```python
from build123d import *

# Parameters (mm, degrees)
BOSS_EXTRUDE1_DEPTH = 2.5
SHELL1_START        = -1.5
SHELL1_DEPTH        = 3
BOSS_EXTRUDE2_START = 2
BOSS_EXTRUDE2_DEPTH = 2
SKETCH4_W           = 30
SKETCH4_H           = 3
CUT_EXTRUDE1_DEPTH  = 100


# Read off the part's stored shape, not the designer's step: Shell1
with BuildPart() as part:
    # Sketch1 → Boss-Extrude1 (new, symmetric)
    with BuildSketch(Plane.XY):
        with BuildLine():
            ThreePointArc((-50.662558564, 50), (-52.076772126, 50.585786438), (-52.662558564, 52))
            Line((-52.662558564, 52), (-52.662558564, 53.937975118))
            ThreePointArc((-52.662558564, 53.937975118), (-52.498112524, 54.732167576), (-52.031816903, 55.395758229))
            ThreePointArc((-52.031816903, 55.395758229), (0, 76), (52.031816903, 55.395758229))
            ThreePointArc((52.031816903, 55.395758229), (52.498112524, 54.732167576), (52.662558564, 53.937975118))
            Line((52.662558564, 53.937975118), (52.662558564, 52))
            ThreePointArc((52.662558564, 52), (52.076772126, 50.585786438), (50.662558564, 50))
            Line((50.662558564, 50), (48.989794856, 50))
            ThreePointArc((48.989794856, 50), (0, 70), (-48.989794856, 50))
            Line((-48.989794856, 50), (-50.662558564, 50))
        make_face()
        with BuildLine():
            ThreePointArc((4.302180061, 56), (5.456880599, 55.632993162), (6.187798144, 54.666666667))
            ThreePointArc((6.187798144, 54.666666667), (8.029260752, 52.496291392), (10.847853752, 52.1))
            ThreePointArc((10.847853752, 52.1), (15.425940788, 52.068491802), (19.510205144, 50))
            Line((19.510205144, 50), (24.864501465, 50))
            ThreePointArc((24.864501465, 50), (25.78632175, 50.22510638), (26.500634408, 50.849752638))
            ThreePointArc((26.500634408, 50.849752638), (31, 53.186572392), (35.499365592, 50.849752638))
            ThreePointArc((35.499365592, 50.849752638), (36.21367825, 50.22510638), (37.135498535, 50))
            Line((37.135498535, 50), (48.989794856, 50))
            ThreePointArc((48.989794856, 50), (0, 70), (-48.989794856, 50))
            Line((-48.989794856, 50), (-37.135498535, 50))
            ThreePointArc((-37.135498535, 50), (-36.21367825, 50.22510638), (-35.499365592, 50.849752638))
            ThreePointArc((-35.499365592, 50.849752638), (-31, 53.186572392), (-26.500634408, 50.849752638))
            ThreePointArc((-26.500634408, 50.849752638), (-25.78632175, 50.22510638), (-24.864501465, 50))
            Line((-24.864501465, 50), (-19.510205144, 50))
            ThreePointArc((-19.510205144, 50), (-15.425940788, 52.068491802), (-10.847853752, 52.1))
            ThreePointArc((-10.847853752, 52.1), (-8.029260752, 52.496291392), (-6.187798144, 54.666666667))
            ThreePointArc((-6.187798144, 54.666666667), (-5.456880599, 55.632993162), (-4.302180061, 56))
            Line((-4.302180061, 56), (4.302180061, 56))
        make_face()
    extrude(amount=BOSS_EXTRUDE1_DEPTH, both=True)

    # Shell1 outline → Shell1 (cut)
    with BuildSketch(Plane.XY.offset(SHELL1_START)):
        with BuildLine():
            Line((37.135498535, 50), (50.662558564, 50))
            Line((50.662558564, 50), (50.662558564, 51))
            ThreePointArc((50.662558564, 51), (51.369665345, 51.292893219), (51.662558564, 52))
            Line((51.662558564, 52), (51.662558564, 53.937975118))
            ThreePointArc((51.662558564, 53.937975118), (51.580335544, 54.335071347), (51.347187733, 54.666866673))
            ThreePointArc((51.347187733, 54.666866673), (0, 75), (-51.347187733, 54.666866673))
            ThreePointArc((-51.347187733, 54.666866673), (-51.580335544, 54.335071347), (-51.662558564, 53.937975118))
            Line((-51.662558564, 53.937975118), (-51.662558564, 52))
            ThreePointArc((-51.662558564, 52), (-51.369665345, 51.292893219), (-50.662558564, 51))
            Line((-50.662558564, 51), (-50.662558564, 50))
            Line((-50.662558564, 50), (-37.135498535, 50))
            ThreePointArc((-37.135498535, 50), (-36.21367825, 50.22510638), (-35.499365592, 50.849752638))
            ThreePointArc((-35.499365592, 50.849752638), (-31, 53.186572392), (-26.500634408, 50.849752638))
            ThreePointArc((-26.500634408, 50.849752638), (-25.78632175, 50.22510638), (-24.864501465, 50))
            Line((-24.864501465, 50), (-19.510205144, 50))
            ThreePointArc((-19.510205144, 50), (-15.425940787, 52.068491802), (-10.847853752, 52.1))
            ThreePointArc((-10.847853752, 52.1), (-8.029260752, 52.496291392), (-6.187798144, 54.666666667))
            ThreePointArc((-6.187798144, 54.666666667), (-5.456880599, 55.632993162), (-4.302180061, 56))
            Line((-4.302180061, 56), (4.302180061, 56))
            ThreePointArc((4.302180061, 56), (5.456880599, 55.632993162), (6.187798144, 54.666666667))
            ThreePointArc((6.187798144, 54.666666667), (8.029260752, 52.496291392), (10.847853752, 52.1))
            ThreePointArc((10.847853752, 52.1), (15.425940787, 52.068491802), (19.510205144, 50))
            Line((19.510205144, 50), (24.864501465, 50))
            ThreePointArc((24.864501465, 50), (25.78632175, 50.22510638), (26.500634408, 50.849752638))
            ThreePointArc((26.500634408, 50.849752638), (31, 53.186572392), (35.499365592, 50.849752638))
            ThreePointArc((35.499365592, 50.849752638), (36.21367825, 50.22510638), (37.135498535, 50))
        make_face()
    extrude(amount=SHELL1_DEPTH, mode=Mode.SUBTRACT)

    # Sketch3 → Boss-Extrude2 (add)
    with BuildSketch(Plane.XY.offset(2.5).offset(BOSS_EXTRUDE2_START)):
        with BuildLine():
            ThreePointArc((48.989794856, 50), (0, 70), (-48.989794856, 50))
            Line((-48.989794856, 50), (-37.135498535, 50))
            ThreePointArc((-37.135498535, 50), (-36.21367825, 50.22510638), (-35.499365592, 50.849752638))
            ThreePointArc((-35.499365592, 50.849752638), (-31, 53.186572392), (-26.500634408, 50.849752638))
            ThreePointArc((-26.500634408, 50.849752638), (-25.78632175, 50.22510638), (-24.864501465, 50))
            Line((-24.864501465, 50), (-19.510205144, 50))
            ThreePointArc((-19.510205144, 50), (-15.425940788, 52.068491802), (-10.847853752, 52.1))
            ThreePointArc((-10.847853752, 52.1), (-8.029260752, 52.496291392), (-6.187798144, 54.666666667))
            ThreePointArc((-6.187798144, 54.666666667), (-5.456880599, 55.632993162), (-4.302180061, 56))
            Line((-4.302180061, 56), (4.302180061, 56))
            ThreePointArc((4.302180061, 56), (5.456880599, 55.632993162), (6.187798144, 54.666666667))
            ThreePointArc((6.187798144, 54.666666667), (8.029260752, 52.496291392), (10.847853752, 52.1))
            ThreePointArc((10.847853752, 52.1), (15.425940788, 52.068491802), (19.510205144, 50))
            Line((19.510205144, 50), (24.864501465, 50))
            ThreePointArc((24.864501465, 50), (25.78632175, 50.22510638), (26.500634408, 50.849752638))
            ThreePointArc((26.500634408, 50.849752638), (31, 53.186572392), (35.499365592, 50.849752638))
            ThreePointArc((35.499365592, 50.849752638), (36.21367825, 50.22510638), (37.135498535, 50))
            Line((37.135498535, 50), (48.989794856, 50))
        make_face()
    extrude(amount=-BOSS_EXTRUDE2_DEPTH)

    # Sketch4 → Cut-Extrude1 (cut, symmetric)
    with BuildSketch(Plane(origin=(0, 0, 0), x_dir=(1, 0, 0), z_dir=(0, 1, 0))):
        with Locations((-20, 0)):
            Rectangle(SKETCH4_W, SKETCH4_H)
        with Locations((20, 0)):
            Rectangle(SKETCH4_W, SKETCH4_H)
    extrude(amount=CUT_EXTRUDE1_DEPTH, both=True, mode=Mode.SUBTRACT)


solid = part.part
```
The model under review builds one solid part; all positions refer to its coordinate system, in mm. A direction names the side the tool comes from. Coordinates: 2 decimals unless noted, no trailing zeros. Write each loop counter-clockwise with the first axis right and the second up, starting at its lowest first coordinate (ties: lowest second). Pieces come first, ordered by that corner, then holes. Notation, with made-up numbers: (16.25, 54) -> (55.25, 54) arc R15 ccw to (55.25, 58) -> close; hole circle Ø3 at (-32.75, -17). An arc over 180 degrees is marked (long way). One line per item, written item: value. Start each with the question number.
Q1. For faces 4 (the face through (0.76, 69.996, 3.514)), 5 (the face through (-44, 50, 3)), 6 (the face through (0, 56, 3)), 7 (the face through (-51.663, 53, 0)), 8 (the face through (-52.663, 53, 0)), list the 3-axis set-ups (+Z, -Z, +X, -X, +Y, -Y) from which the entire face can be reached by the end or side of a thin tool; tool diameter is ignored.
Q2. Add section B-B, the plane y = 68.75. Give the boundary of the cut face in (x, z).
Q3. The part is to be moulded in two halves that separate along Z. For faces 1 (the face through (52.09, 50.6, 0.04)), 2 (the face through (51.663, 53, 0)), 3 (the face through (-1, 60, 4.5)), say which applies: +Z half, -Z half, draft (parallel to the pull), parting line (faces both ways), or undercut.
Q4. Add section A-A, the plane z = -0.5. Give the boundary of the cut face in (x, y), then the cut area to 3 significant figures.
Q5. Add section D-D, the plane z = 3.5. Give the boundary of the cut face in (x, y), then the cut area to 3 significant figures.
Q6. Add section C-C, the plane x = 31. Give the boundary of the cut face in (y, z).
Q7. To check wall thickness, follow probe 1 along Z at (x, y) = (-27.5, 68); probe 2 along Z at (x, y) = (-16, 58.25); probe 3 along X at (y, z) = (61.75, -0.5). State the ranges of each line that lie inside material, in increasing order.
Q8. Clearance check with flat-ended pins moving along their axes: P1, Ø3, axis at x = 37, y = 70, coming from the -Z side; P2, Ø0.8, axis at y = 50.5, z = 0.5, coming from the -X side; P3, Ø0.8, axis at y = 75.5, z = 0, coming from the -X side; P4, Ø0.6, axis at y = 66.5, z = 0.5, coming from the +X side. State where each tip first meets the part, or that it passes through.
Response:
1. face 4: +Z, +Y
1. face 5: +Z, -Z, +X, -X, -Y
1. face 6: +Z, -Z, -Y
1. face 7: none
1. face 8: +Z, -Z, -X, +Y, -Y
2. outline: (-32.4, -2.5) -> (32.4, -2.5) -> (32.4, -1.5) -> (-32.4, -1.5) -> close; (-32.4, 1.5) -> (32.4, 1.5) -> (32.4, 2.5) -> (13.17, 2.5) -> (13.17, 4.5) -> (-13.17, 4.5) -> (-13.17, 2.5) -> (-32.4, 2.5) -> close
3. face 1: draft
3. face 2: undercut
3. face 3: +Z half
4. outline: (-52.66, 52) arc R2 ccw to (-50.66, 50) -> (-50.66, 51) arc R1 cw to (-51.66, 52) -> (-51.66, 53.94) arc R1 cw to (-51.35, 54.67) arc R75 cw to (-35, 66.33) -> (-35, 67.46) arc R76 ccw to (-52.03, 55.4) arc R2 ccw to (-52.66, 53.94) -> close; (-5, 74.83) arc R75 cw to (5, 74.83) -> (5, 75.84) arc R76 ccw to (-5, 75.84) -> close; (35, 66.33) arc R75 cw to (51.35, 54.67) arc R1 cw to (51.66, 53.94) -> (51.66, 52) arc R1 cw to (50.66, 51) -> (50.66, 50) arc R2 ccw to (52.66, 52) -> (52.66, 53.94) arc R2 ccw to (52.03, 55.4) arc R76 ccw to (35, 67.46) -> close
4. area: 62.1 mm²
5. outline: (-48.99, 50) -> (-37.14, 50) arc R2 ccw to (-35.5, 50.85) arc R5.5 cw to (-26.5, 50.85) arc R2 ccw to (-24.86, 50) -> (-19.51, 50) arc R10 cw to (-10.85, 52.1) arc R4 ccw to (-6.19, 54.67) arc R2 cw to (-4.3, 56) -> (4.3, 56) arc R2 cw to (6.19, 54.67) arc R4 ccw to (10.85, 52.1) arc R10 cw to (19.51, 50) -> (24.86, 50) arc R2 ccw to (26.5, 50.85) arc R5.5 cw to (35.5, 50.85) arc R2 ccw to (37.14, 50) -> (48.99, 50) arc R70 ccw to start
5. area: 1,170 mm²
6. outline: (53.19, -2.5) -> (69.39, -2.5) -> (69.39, -1.5) -> (53.19, -1.5) -> close; (53.19, 1.5) -> (69.39, 1.5) -> (69.39, 2.5) -> (62.76, 2.5) -> (62.76, 4.5) -> (53.19, 4.5) -> close
7. probe 1: -2.5 to -1.5, 1.5 to 2.5
7. probe 2: -2.5 to -1.5, 1.5 to 4.5
7. probe 3: -44.31 to -42.57, 42.57 to 44.31
8. P1: through
8. P2: x = -52.33
8. P3: x = -5
8. P4: x = 37.33
